```python
from build123d import *

# Parameters (mm, degrees)
PAD_DEPTH       = 10
SKETCH001_W     = 100
SKETCH001_H     = 6
PAD001_DEPTH    = 19
POCKET_DEPTH    = 25.001
SKETCH003_W     = 59.99999
SKETCH003_H     = 15.5
POCKET001_DEPTH = 25.001
SKETCH004_R     = 2
POCKET002_DEPTH = 25.001
SKETCH005_R     = 3
POCKET003_DEPTH = 3.5
FILLET_R        = 3.9
FILLET001_R     = 30
SKETCH006_R     = 2
POCKET004_DEPTH = 10.001
CHAMFER_SIZE    = 19
FILLET002_R     = 10
CHAMFER001_SIZE = 2
CHAMFER002_SIZE = 3
CHAMFER003_SIZE = 3
CHAMFER004_SIZE = 0.5
PAD002_DEPTH    = 2.5


with BuildPart() as part:
    # Sketch → Pad (new body)
    with BuildSketch(Plane.XY):
        Polygon((50, -22.05), (25, 26.05), (-25, 26.05), (-50, -22.05), (-50, -47.05), (50, -47.05), align=None)
        with BuildLine():
            ThreePointArc((-7.5, 16.05), (-23.55, 0), (-7.5, -16.05))
            Line((-7.5, -16.05), (7.5, -16.05))
            ThreePointArc((7.5, -16.05), (23.55, 0), (7.5, 16.05))
            Line((-7.5, 16.05), (7.5, 16.05))
        make_face(mode=Mode.SUBTRACT)
    extrude(amount=PAD_DEPTH)

    # Sketch001 (on Face12 of Pad) → Pad001 (join)
    with BuildSketch(Plane.XY.offset(10)):
        with Locations((0, -25.05)):
            Rectangle(SKETCH001_W, SKETCH001_H)
    extrude(amount=PAD001_DEPTH)

    # Sketch002 (on Face12 of Pad001) → Pocket (cut, through all)
    with BuildSketch(Plane(origin=(0, -22.05, 0), x_dir=(-1, 0, 0), z_dir=(0, 1, 0))):
        with BuildLine():
            ThreePointArc((-50, 13.5), (-45.757359, 15.257359), (-44, 19.5))
            Line((-44, 29), (-44, 19.5))
            Line((-50, 29), (-44, 29))
            Line((-50, 13.5), (-50, 29))
        make_face()
        with BuildLine():
            ThreePointArc((-36, 19.5), (-30, 13.5), (-24, 19.5))
            Line((-24, 29), (-24, 19.5))
            Line((-36, 29), (-24, 29))
            Line((-36, 19.5), (-36, 29))
        make_face()
        with BuildLine():
            ThreePointArc((-16, 19.5), (-10, 13.5), (-4, 19.5))
            Line((-4, 29), (-4, 19.5))
            Line((-16, 29), (-4, 29))
            Line((-16, 19.5), (-16, 29))
        make_face()
        with BuildLine():
            ThreePointArc((4, 19.5), (10, 13.5), (16, 19.5))
            Line((16, 29), (16, 19.5))
            Line((4, 29), (16, 29))
            Line((4, 19.5), (4, 29))
        make_face()
        with BuildLine():
            ThreePointArc((24, 19.5), (30, 13.5), (36, 19.5))
            Line((36, 29), (36, 19.5))
            Line((24, 29), (36, 29))
            Line((24, 19.5), (24, 29))
        make_face()
        with BuildLine():
            ThreePointArc((44, 19.5), (45.757359, 15.257359), (50, 13.5))
            Line((50, 29), (50, 13.5))
            Line((44, 29), (50, 29))
            Line((44, 19.5), (44, 29))
        make_face()
    extrude(amount=-POCKET_DEPTH, mode=Mode.SUBTRACT)

    # Sketch003 (on Face10 of Pocket) → Pocket001 (cut, through all)
    with BuildSketch(Plane(origin=(0, -22.05, 0), x_dir=(-1, 0, 0), z_dir=(0, 1, 0))):
        with Locations((-5e-06, 21.25)):
            Rectangle(SKETCH003_W, SKETCH003_H)
    extrude(amount=-POCKET001_DEPTH, mode=Mode.SUBTRACT)

    # Sketch004 (on Face10 of Pocket001) → Pocket002 (cut, through all)
    with BuildSketch(Plane(origin=(0, -22.05, 0), x_dir=(-1, 0, 0), z_dir=(0, 1, 0))):
        with Locations((-40, 25)):
            Circle(SKETCH004_R)
        with Locations((40, 25)):
            Circle(SKETCH004_R)
    extrude(amount=-POCKET002_DEPTH, mode=Mode.SUBTRACT)

    # Sketch005 (on Face10 of Pocket002) → Pocket003 (cut)
    with BuildSketch(Plane(origin=(0, -22.05, 0), x_dir=(-1, 0, 0), z_dir=(0, 1, 0))):
        with Locations((-40, 25)):
            Circle(SKETCH005_R)
        with Locations((40, 25)):
            Circle(SKETCH005_R)
    extrude(amount=-POCKET003_DEPTH, mode=Mode.SUBTRACT)

    # Fillet
    fillet_edges = [part.edges().sort_by_distance(p)[0] for p in [
        (36, -25.05, 29),
        (44, -25.05, 29),
        (-36, -25.05, 29),
        (-44, -25.05, 29),
    ]]
    fillet(fillet_edges, radius=FILLET_R)

    # Fillet001
    fillet001_edges = [part.edges().sort_by_distance(p)[0] for p in [
        (25, 26.05, 5),
        (-25, 26.05, 5),
    ]]
    fillet(fillet001_edges, radius=FILLET001_R)

    # Sketch006 (on Face15 of Fillet001) → Pocket004 (cut, through all)
    with BuildSketch(Plane.XY.offset(10)):
        with Locations((-20, -38.05)):
            Circle(SKETCH006_R)
        with Locations((20, -38.05)):
            Circle(SKETCH006_R)
    extrude(amount=-POCKET004_DEPTH, mode=Mode.SUBTRACT)

    # Chamfer
    chamfer_edges = [part.edges().sort_by_distance(p)[0] for p in [
        (-50, -47.05, 5),
        (50, -47.05, 5),
    ]]
    chamfer(chamfer_edges, length=CHAMFER_SIZE)

    # Fillet002
    fillet002_edges = [part.edges().sort_by_distance(p)[0] for p in [
        (-31, -47.05, 5),
        (31, -47.05, 5),
    ]]
    fillet(fillet002_edges, radius=FILLET002_R)

    # Chamfer001
    chamfer001_edges = [part.edges().sort_by_distance(p)[0] for p in [
        (-41.700791, -6.082323, 0),
        (-50, -25.05, 0),
        (-41.964466, -36.085534, 0),
        (50, -25.05, 0),
        (-41.700791, -6.082323, 10),
        (-41.964466, -36.085534, 10),
    ]]
    chamfer(chamfer001_edges, length=CHAMFER001_SIZE)

    # Chamfer002
    chamfer002_edges = [part.edges().sort_by_distance(p)[0] for p in [
        (-50, -25.05, 13.5),
        (50, -25.05, 13.5),
    ]]
    chamfer(chamfer002_edges, length=CHAMFER002_SIZE)

    # Chamfer003
    chamfer003_edges = [part.edges().sort_by_distance(p)[0] for p in [
        (0, -22.05, 10),
    ]]
    chamfer(chamfer003_edges, length=CHAMFER003_SIZE)

    # Chamfer004
    chamfer004_edges = [part.edges().sort_by_distance(p)[0] for p in [
        (-23.55, 0, 0),
        (-23.55, 0, 10),
    ]]
    chamfer(chamfer004_edges, length=CHAMFER004_SIZE)

    # Sketch007 → Pad002 (join, symmetric)
    with BuildSketch(Plane.YZ.offset(-40)):
        Polygon((-22.05, 20), (-22.05, 10), (-12.05, 10), align=None)
    pad002 = extrude(amount=PAD002_DEPTH, both=True)

    # Mirrored: Pad002 across YZ
    add(pad002.mirror(Plane.YZ))


solid = part.part
```
Source: CAD feature listing. Evaluate the final solid. Frame: model axes, mm. A direction names the side the tool comes from. Give positions to 0.01 mm unless a question says otherwise; leave off trailing zeros. Order: outer loops, then holes, each group sorted by start corner. A loop starts at its lowest first (then second) coordinate and runs counter-clockwise, first axis right, second up.
(1) Section query D-D (y = -30.5). Return the cut outline in (x, z), plus the area to 3 significant figures.
(2) Pull-direction query (X, two-part tool) for faces 4 (the face through (30.18, -45.19, 0.79)), 5 (the face through (-21.31, 20.391, 0.347)), 6 (the face through (0, -25, 13.5)), 7 (the face through (0, -17, 10)); classes: +X half, -X half, draft (parallel to the pull), parting line (faces both ways), or undercut.
(3) Section query A-A (x = 4.5). Return the cut outline in (y, z), plus the area to 3 significant figures.
(4) Section query B-B (z = 3.75). Return the cut outline in (x, y), plus the area to 3 significant figures.
(5) Material intervals for line 1 along Z through (x, y) = (40, -23.35); line 2 along Z through (x, y) = (40, -26.95); line 3 along Y through (x, z) = (-20, 6.25), sorted ascending.
(6) Access query for faces 1 (the face through (44.854, -25.008, 16.414)), 2 (the face through (-43.96, -20.53, 11.48)), 3 (the face through (43, -24, 25)). Directions: +Z, -Z, +X, -X, +Y, -Y. A direction counts if a zero-diameter tool reaches every point of the face in a straight line with its end or side. Return the directions, or none.
(7) Contact query for flat-ended pins moving along their axis: P1, Ø2, axis at x = 27, z = 15, coming from the -Y side; P2, Ø3, axis at y = -24.5, z = 22.5, coming from the -X side; P3, Ø3, axis at x = 36, z = 25, coming from the +Y side; P4, Ø6.5, axis at x = -23.5, z = 14, coming from the +Y side. Output: stop coordinate, or through.
(8) Section query C-C (y = -38.05). Return the cut outline in (x, z), plus the area to 3 significant figures.
Outcome:
1. outline: (-47.55, 2) - (-44.72, 0) - (44.72, 0) - (47.55, 2) - (47.55, 8) - (44.72, 10) - (-44.72, 10) - (-47.55, 8) - close
1. area: 940 mm2
2. face 4: +X half
2. face 5: -X half
2. face 6: undercut
2. face 7: undercut
3. outline: (-47.05, 2) - (-45.05, 0) - (-16.55, 0) - (-16.05, 0.5) - (-16.05, 9.5) - (-16.55, 10) - (-19.05, 10) - (-22.05, 13) - (-22.05, 13.5) - (-28.05, 13.5) - (-28.05, 10) - (-45.05, 10) - (-47.05, 8) - close; (16.05, 0.5) - (16.55, 0) - (24.05, 0) - (26.05, 2) - (26.05, 8) - (24.05, 10) - (16.55, 10) - (16.05, 9.5) - close
3. area: 427 mm2
4. outline: (-50, -28.05) - (-33.93, -44.12) arc R10 ccw to (-26.86, -47.05) - (26.86, -47.05) arc R10 ccw to (33.93, -44.12) - (50, -28.05) - (50, -22.05) - (33.4, 9.89) arc R30 ccw to (6.78, 26.05) - (-6.78, 26.05) arc R30 ccw to (-33.4, 9.89) - (-50, -22.05) - close; hole circle Ø4 at (-20, -38.05); hole (-7.5, -16.05) - (7.5, -16.05) arc R16.05 ccw to (7.5, 16.05) - (-7.5, 16.05) arc R16.05 ccw to start; hole circle Ø4 at (20, -38.05)
4. area: 4,320 mm2
5. line 1: z = 0 to 22, 28 to 29
5. line 2: z = 0 to 23, 27 to 29
5. line 3: y = -47.05 to -40.05, -36.05 to -10.07, 10.07 to 22.98
6. face 1: +Z, +X, +Y, -Y
6. face 2: +Z, -X, +Y
6. face 3: +Y
7. P1: passes through
7. P2: stops at x = -44
7. P3: stops at y = -22.05
7. P4: stops at y = -19.8
8. outline: (-40, 2) - (-37.17, 0) - (-22, 0) - (-22, 10) - (-37.17, 10) - (-40, 8) - close; (-18, 0) - (18, 0) - (18, 10) - (-18, 10) - close; (22, 0) - (37.17, 0) - (40, 2) - (40, 8) - (37.17, 10) - (22, 10) - close
8. area: 709 mm2
